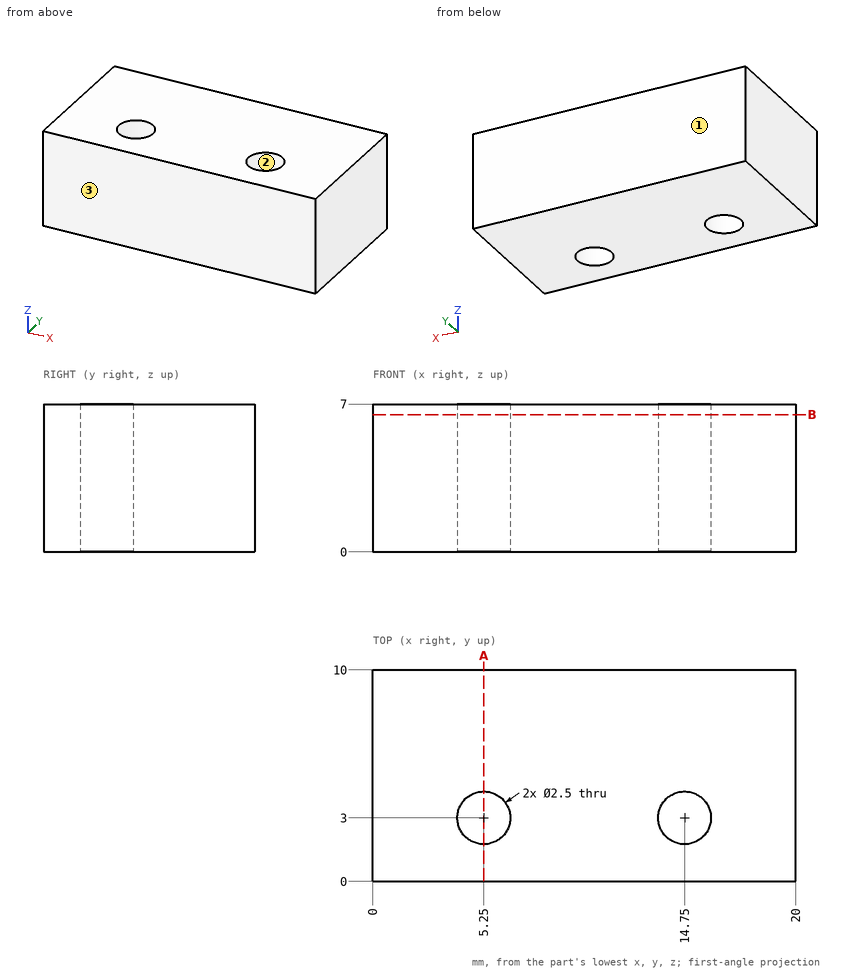
Verification items for this drawing (mm, ordinates from the low corner). Round coordinates to 2 decimals unless told otherwise and drop trailing zeros. Order: outer loops, then holes, each group sorted by start corner. A loop starts at its lowest first (then second) coordinate and runs counter-clockwise, first axis right, second up. Notation, with made-up numbers: M -6,55.25 L 1,55.25 A18 ccw 1,60.25 Z; hole C 83,73 d1. An arc over 180 degrees is marked long. Answer in a Markdown table with one row per item. Add a question column.
Item 1: Sectioned sample at A-A, the plane x = 5.25. Enter the section's corners in (y, z).
Item 2: Sectioned sample at B-B, the plane z = 6.5. Enter the section's corners in (x, y), plus the area to 3 significant figures.
Item 3: Material ranges on L1, parallel to X at y = 4, z = 6; L2, parallel to Y at x = 5.25, z = 2.5; L3, parallel to Y at x = 4.5, z = 2, recorded low to high. Write a range as [from, to].
Item 4: Draft check along Y on the marked faces 1, 2 and 3. Enter one of: released by +Y, released by -Y, zero draft, split by the parting line, or undercut.
Filled in:
| question | item | result |
|---|---|---|
| 1 | outline | M 0,0 L 1.75,0 L 1.75,7 L 0,7 Z; M 4.25,0 L 10,0 L 10,7 L 4.25,7 Z |
| 2 | outline | M 0,0 L 20,0 L 20,10 L 0,10 Z; hole C 5.25,3 d2.5; hole C 14.75,3 d2.5 |
| 2 | area | 190 mm² |
| 3 | L1 | x = [0, 4.5], [6, 14], [15.5, 20] |
| 3 | L2 | y = [0, 1.75], [4.25, 10] |
| 3 | L3 | y = [0, 2], [4, 10] |
| 4 | face 1 | released by +Y |
| 4 | face 2 | undercut |
| 4 | face 3 | released by -Y |
